from build123d import *

# Parameters (mm, degrees)
F1_DEPTH = 203.2
F3_DEPTH = 25.4


# Not quite as in the source:
# - ends of sketch curves that miss each other by under 0.0002 mm in the source are joined


with BuildPart() as f1:
    # F0 (on Top) → F1 (new body)
    with BuildSketch(Plane.XY):
        with BuildLine():
            Line((0, -6.35), (0, -63.5))
            Line((0, -63.5), (6.35, -63.5))
            Line((6.35, -63.5), (6.35, -9.525))
            ThreePointArc((6.35, -9.525), (7.2799359697, -7.2799359697), (9.525, -6.35))
            Line((9.525, -6.35), (63.5, -6.35))
            Line((63.5, -6.35), (63.5, 0))
            Line((63.5, 0), (6.35, 0))
            Line((6.35, 0), (0, 0))
            Line((0, 0), (0, -6.35))
        make_face()
    extrude(amount=F1_DEPTH)

    # F2 (on face) → F3 (cut)
    with BuildSketch(Plane.XZ.offset(6.35)):
        with BuildLine():
            Line((38.1, 165.8788350046), (63.5, 165.8788350046))
            Line((63.5, 165.8788350046), (63.5, 176.9913350046))
            Line((63.5, 176.9913350046), (38.1, 176.9913350046))
            ThreePointArc((38.1, 176.9913350046), (32.54375, 171.4350850046), (38.1, 165.8788350046))
        make_face()
        with BuildLine():
            Line((34.925, 37.2913350046), (34.8918574917, 37.2913350046))
            ThreePointArc((34.8918574917, 37.2913350046), (29.3687747109, 31.7185139715), (34.925, 26.1788350046))
            Line((34.925, 26.1788350046), (63.5, 26.1788350046))
            Line((63.5, 26.1788350046), (63.5, 37.2913350046))
            Line((63.5, 37.2913350046), (34.925, 37.2913350046))
        make_face()
    extrude(amount=-F3_DEPTH, mode=Mode.SUBTRACT)


solid = f1.part
Check sheet for the modelled part. Datum: model origin and axes. Units: mm. A direction names the side the tool comes from. Give positions to 0.01 mm unless a question says otherwise; leave off trailing zeros. Write each loop counter-clockwise with the first axis right and the second up, starting at its lowest first coordinate (ties: lowest second). Pieces come first, ordered by that corner, then holes. Notation, with made-up numbers: M 25.25,-0.5 L 50.25,-0.5 A24 ccw 50.25,19.5 Z; hole C -40,-28 d3. An arc over 180 degrees is marked long. Use one line per item in the form item = value.
(1) Section check C-C on x = 27.5. Record the boundary of the cut face in (y, z).
Answer block:
outline = M -6.35,0 L 0,0 L 0,203.2 L -6.35,203.2 Z
(2) Draft check along Z on faces 4 (the flat face through (63.5, -3, 101)), 5 (the flat face through (51, -3, 165.879)), 6 (the flat face through (6, -17, 0)). Enter one of: pulls with the +Z half, pulls with the -Z half, needs draft (parallel to the pull), parting line crosses it, or undercut.
Answer block:
face_4 = needs draft
face_5 = undercut
face_6 = pulls with the -Z half
(3) Depth check by flat-ended pin: P1, Ø10, axis at x = 35, z = 45.5, coming from the -Y side; P2, Ø1, axis at y = -47.5, z = 133.5, coming from the +X side. Enter the tip coordinate at first touch or a pass-through.
Answer block:
P1 = -6.35
P2 = 6.35
(4) Tool access check on faces 1 (the flat face through (49, -3, 26.179)), 2 (the flat face through (63.5, -3, 13)), 3 (the flat face through (6.35, -37, 100)). Record the directions out of +Z, -Z, +X, -X, +Y, -Y that give a thin tool (end or side, any length) a straight path to the whole face; none if there is none.
Answer block:
face_1 = +X, +Y, -Y
face_2 = +Z, -Z, +X, +Y, -Y
face_3 = +Z, -Z, +X, -Y
(5) Section check D-D on y = -47.5. Record the boundary of the cut face in (x, z), plus the area to 3 significant figures.
Answer block:
outline = M 0,0 L 6.35,0 L 6.35,203.2 L 0,203.2 Z
area = 1,290 mm2
(6) Section check B-B on z = 137. Record the boundary of the cut face in (x, y) (3 decimals), plus the area to 3 significant figures.
Answer block:
outline = M 0,-63.5 L 6.35,-63.5 L 6.35,-9.525 A3.175 cw 9.525,-6.35 L 63.5,-6.35 L 63.5,0 L 0,0 Z
area = 768 mm2
(7) Material ranges on line 1 along Y through (x, z) = (38.5, 72.5); line 2 along X through (y, z) = (-54, 26.5), recorded low to high.
Answer block:
line_1 = -6.35 to 0
line_2 = 0 to 6.35
(8) Section check A-A on x = 51. Record the boundary of the cut face in (y, z), plus the area to 3 significant figures.
Answer block:
outline = M -6.35,0 L 0,0 L 0,26.18 L -6.35,26.18 Z; M -6.35,37.29 L 0,37.29 L 0,165.88 L -6.35,165.88 Z; M -6.35,176.99 L 0,176.99 L 0,203.2 L -6.35,203.2 Z
area = 1,150 mm2
